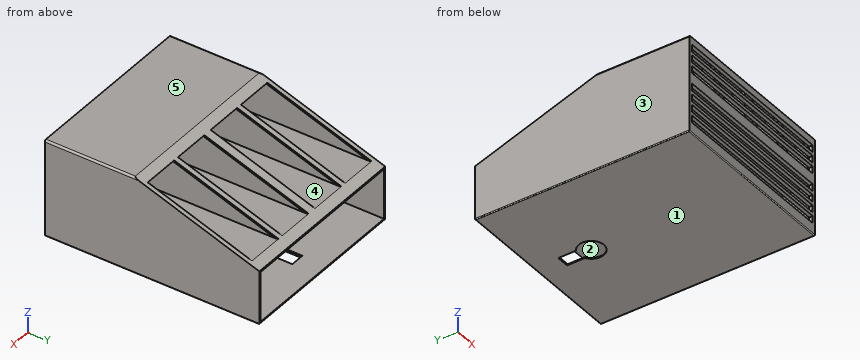
```python
from build123d import *

# Parameters (mm, degrees)
SKETCH_W        = 100
SKETCH_H        = 120
PAD_DEPTH       = 30
SKETCH001_W     = 98
SKETCH001_H     = 28
POCKET_DEPTH    = 118
POCKET006_DEPTH = 2
PAD001_DEPTH    = 100
SKETCH012_W     = 20
SKETCH012_H     = 20
POCKET011_DEPTH = 118
SKETCH016_W     = 96
SKETCH016_H     = 4
POCKET012_DEPTH = 2
SKETCH014_W     = 96
SKETCH014_H     = 4
POCKET013_DEPTH = 2
SKETCH013_W     = 96
SKETCH013_H     = 4
POCKET014_DEPTH = 2
SKETCH009_W     = 96
SKETCH009_H     = 4
POCKET015_DEPTH = 2
SKETCH003_W     = 96
SKETCH003_H     = 4
POCKET016_DEPTH = 2
SKETCH007_W     = 96
SKETCH007_H     = 4
POCKET017_DEPTH = 2
SKETCH008_W     = 96
SKETCH008_H     = 4
POCKET018_DEPTH = 2
FILLET_R        = 0.5
FILLET001_R     = 1
FILLET002_R     = 1
CHAMFER_SIZE    = 0.5
CHAMFER001_SIZE = 0.5


with BuildPart() as part:
    # Sketch → Pad (new body)
    with BuildSketch(Plane.XY):
        Rectangle(SKETCH_W, SKETCH_H)
    extrude(amount=PAD_DEPTH)

    # Sketch001 → Pocket (cut)
    with BuildSketch(Plane.XZ.offset(58)):
        with Locations((0, 15)):
            Rectangle(SKETCH001_W, SKETCH001_H)
    extrude(amount=-POCKET_DEPTH, mode=Mode.SUBTRACT)

    # Sketch010 → Pocket006 (cut)
    with BuildSketch(Plane.XY):
        with BuildLine():
            Line((-3.5, 46.062178), (3.5, 46.062178))
            Line((3.5, 46.062178), (3.5, 36.062178))
            ThreePointArc((-3.5, 36.062178), (0, 23), (3.5, 36.062178))
            Line((-3.5, 36.062178), (-3.5, 46.062178))
        make_face()
    extrude(amount=POCKET006_DEPTH, mode=Mode.SUBTRACT)

    # Sketch011 → Pad001 (join)
    with BuildSketch(Plane.YZ.offset(50)):
        Polygon((60, 30), (-60, 30), (-60, 54), (-10, 54), align=None)
    extrude(amount=-PAD001_DEPTH)

    # Sketch012 → Pocket011 (cut)
    with BuildSketch(Plane.XZ.offset(58)):
        with Locations((37, 42)):
            Rectangle(SKETCH012_W, SKETCH012_H)
        with Locations((13, 42)):
            Rectangle(SKETCH012_W, SKETCH012_H)
        with Locations((-13, 42)):
            Rectangle(SKETCH012_W, SKETCH012_H)
        with Locations((-37, 42)):
            Rectangle(SKETCH012_W, SKETCH012_H)
    extrude(amount=-POCKET011_DEPTH, mode=Mode.SUBTRACT)

    # Sketch016 → Pocket012 (cut)
    with BuildSketch(Plane.XZ.offset(60)):
        with Locations((0, 48)):
            Rectangle(SKETCH016_W, SKETCH016_H)
    extrude(amount=-POCKET012_DEPTH, mode=Mode.SUBTRACT)

    # Sketch014 → Pocket013 (cut)
    with BuildSketch(Plane.XZ.offset(60)):
        with Locations((0, 42)):
            Rectangle(SKETCH014_W, SKETCH014_H)
    extrude(amount=-POCKET013_DEPTH, mode=Mode.SUBTRACT)

    # Sketch013 → Pocket014 (cut)
    with BuildSketch(Plane.XZ.offset(60)):
        with Locations((0, 36)):
            Rectangle(SKETCH013_W, SKETCH013_H)
    extrude(amount=-POCKET014_DEPTH, mode=Mode.SUBTRACT)

    # Sketch009 → Pocket015 (cut)
    with BuildSketch(Plane.XZ.offset(60)):
        with Locations((0, 26)):
            Rectangle(SKETCH009_W, SKETCH009_H)
    extrude(amount=-POCKET015_DEPTH, mode=Mode.SUBTRACT)

    # Sketch003 → Pocket016 (cut)
    with BuildSketch(Plane.XZ.offset(60)):
        with Locations((0.01379, 20)):
            Rectangle(SKETCH003_W, SKETCH003_H)
    extrude(amount=-POCKET016_DEPTH, mode=Mode.SUBTRACT)

    # Sketch007 → Pocket017 (cut)
    with BuildSketch(Plane.XZ.offset(60)):
        with Locations((0, 14)):
            Rectangle(SKETCH007_W, SKETCH007_H)
    extrude(amount=-POCKET017_DEPTH, mode=Mode.SUBTRACT)

    # Sketch008 → Pocket018 (cut)
    with BuildSketch(Plane.XZ.offset(60)):
        with Locations((0, 8)):
            Rectangle(SKETCH008_W, SKETCH008_H)
    extrude(amount=-POCKET018_DEPTH, mode=Mode.SUBTRACT)

    # Fillet
    fillet_edges = [part.edges().sort_by_distance(p)[0] for p in [
        (0, -60, 0),
        (-50, 0, 0),
        (50, 0, 0),
        (0, 60, 0),
    ]]
    fillet(fillet_edges, radius=FILLET_R)

    # Fillet001
    fillet001_edges = [part.edges().sort_by_distance(p)[0] for p in [
        (50, -35, 54),
    ]]
    fillet(fillet001_edges, radius=FILLET001_R)

    # Fillet002
    fillet002_edges = [part.edges().sort_by_distance(p)[0] for p in [
        (-50, -35, 54),
    ]]
    fillet(fillet002_edges, radius=FILLET002_R)

    # Chamfer
    chamfer_edges = [part.edges().sort_by_distance(p)[0] for p in [
        (47, 25, 42),
        (27, 25, 42),
        (23, 25, 42),
        (3, 25, 42),
        (-3, 25, 42),
        (-23, 25, 42),
        (-27, 25, 42),
        (-47, 25, 42),
    ]]
    chamfer(chamfer_edges, length=CHAMFER_SIZE)

    # Chamfer001
    chamfer001_edges = [part.edges().sort_by_distance(p)[0] for p in [
        (3.5, 41.062178, 1),
        (0, 23, 1),
        (-3.5, 41.062178, 1),
    ]]
    chamfer(chamfer001_edges, length=CHAMFER001_SIZE)


solid = part.part
```
Could you check a few things on this model? Use its own coordinates, in mm. Face numbers are marked on the shaded views. A direction names the side the tool comes from. Give positions to 0.01 mm unless a question says otherwise; leave off trailing zeros. Loops run counter-clockwise (first coordinate to the right, second up) from the corner with the lowest first, then second, coordinate; pieces in that order, holes last. Notation, with made-up numbers: (63, 55) -> (71, 55) arc R22 cw to (71, 71) -> close; hole circle Ø9 at (58.25, 63). An arc over 180 degrees is marked (long way). Put each result on its own line as item: value.
(1) Imagine slicing it at C-C on x = 0. State how many separate pieces and enclosed holes the cut face has, plus the area to 3 significant figures.
Computed:
separate pieces: 6
enclosed holes: 0
area: 2,260 mm^2
(2) I'm going to push flat-ended pins straight in: pin 1 Ø2 at (x, z) = (-39.5, 45) entering from +Y; pin 2 Ø1.2 at (x, z) = (-25.5, 36.5) entering from -Y; pin 3 Ø1.5 at (x, z) = (-18, 26) entering from +Y. Where does each tip first touch, or does it pass through?
Computed:
pin 1: y = -58
pin 2: y = -58
pin 3: through
(3) Imagine slicing it at A-A on z = 20. Write out the boundary of the cut face in (x, y).
Computed:
outline: (-50, -60) -> (-47.99, -60) -> (-47.99, -58) -> (-49, -58) -> (-49, 60) -> (-50, 60) -> close; (48.01, -60) -> (50, -60) -> (50, 60) -> (49, 60) -> (49, -58) -> (48.01, -58) -> close
(4) Please list where these lines run through material, in increasing order: probe 1 along Z at (x, y) = (5, -27); probe 2 along X at (y, z) = (-32.5, 50.5); probe 3 along Z at (x, y) = (15, 14). Write a range as [from, to].
Computed:
probe 1: [0, 1], [29, 32], [52, 54]
probe 2: [-50, -47], [-27, -23], [-3, 3], [23, 27], [47, 50]
probe 3: [0, 1], [29, 32]
(5) Thinking about a two-plate mould opening in Z: for the marked faces 3, 4 and 5, which applies, pulls with the +Z half, pulls with the -Z half, needs draft (parallel to the pull), parting line crosses it, or undercut?
Computed:
face 3: needs draft
face 4: undercut
face 5: pulls with the +Z half
(6) For the marked faces 1 and 2, which set-ups out of +Z, -Z, +X, -X, +Y, -Y let a thin tool reach every point of the face, with its end or its side?
Computed:
face 1: -Z, +X, -X, +Y, -Y
face 2: +Y
(7) Imagine slicing it at B-B on y = -48. Write out the boundary of the cut face in (x, z).
Computed:
outline: (-50, 0.5) arc R0.5 ccw to (-49.5, 0) -> (49.5, 0) arc R0.5 ccw to (50, 0.5) -> (50, 53) arc R1 ccw to (49, 54) -> (-49, 54) arc R1 ccw to (-50, 53) -> close; hole (-49, 1) -> (49, 1) -> (49, 29) -> (-49, 29) -> close; hole (-47, 32) -> (-27, 32) -> (-27, 52) -> (-47, 52) -> close; hole (-23, 32) -> (-3, 32) -> (-3, 52) -> (-23, 52) -> close; hole (3, 32) -> (23, 32) -> (23, 52) -> (3, 52) -> close; hole (27, 32) -> (47, 32) -> (47, 52) -> (27, 52) -> close
